For this review, use the dimensioned drawing (mm, ordinates from the lowest corner) and the shaded views. A direction names the side the tool comes from. Give positions to 0.01 mm unless a question says otherwise; leave off trailing zeros. Write each loop counter-clockwise with the first axis right and the second up, starting at its lowest first coordinate (ties: lowest second). Pieces come first, ordered by that corner, then holes. Notation, with made-up numbers: M 23,6 L 75,6 A35 ccw 75,45 Z; hole C -8,54.25 d2. An arc over 180 degrees is marked long. One line per item, written item: value. Start each with the question number.
Item 1: Clearance check with flat-ended pins moving along their axes: pin 1 Ø2.5 at (x, z) = (11, 29) entering from -Y; pin 2 Ø8 at (y, z) = (8, 21.5) entering from -X; pin 3 Ø1 at (x, y) = (11.5, 10) entering from +Z; pin 4 Ø1.5 at (y, z) = (9.5, 12.5) entering from +X. State where each tip first meets the part, or that it passes through.
Item 2: Consider section A-A, the plane z = 28.5. Write out the cut boundary in (x, y), and give its area (3 significant figures).
Item 3: Consider section C-C, the plane y = 4.5. Write out the cut boundary in (x, z).
Item 4: Consider section D-D, the plane x = 18. Write out the cut boundary in (y, z).
Item 5: Consider section B-B, the plane x = 35. Write out the cut boundary in (y, z), and give its area (3 significant figures).
Item 6: Tool access review of the marked faces 1, 2 and 3: name each direction out of +Z, -Z, +X, -X, +Y, -Y from which nothing blocks a thin tool from reaching the whole face with its end or side.
Item 7: Mouldability with a two-part tool opening along Y and no side actions: class the marked faces 4, 5 and 6 as released by +Y, released by -Y, zero draft, split by the parting line, or undercut.
Item 8: To check wall thickness, follow probe 1 along X at (y, z) = (10, 3.1); probe 2 along Y at (x, z) = (11, 25.5); probe 3 along Z at (x, y) = (16.9, 10). State the ranges of each line that lie inside material, in increasing order.
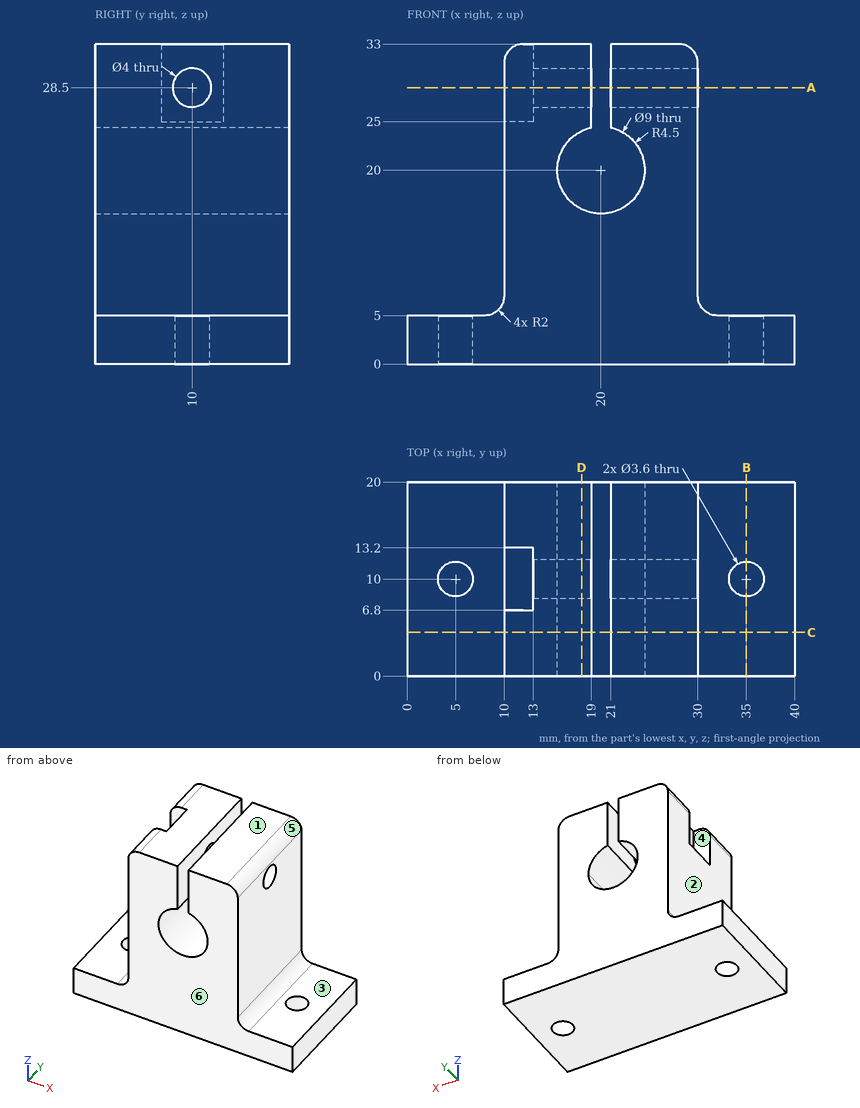
Model answer:
1. pin 1: stops at y = 0
1. pin 2: stops at x = 10
1. pin 3: stops at z = 25
1. pin 4: stops at x = 30
2. outline: M 10,0 L 19,0 L 19,8 L 13,8 L 13,6.8 L 10,6.8 Z; M 10,13.2 L 13,13.2 L 13,12 L 19,12 L 19,20 L 10,20 Z; M 21,0 L 30,0 L 30,8 L 21,8 Z; M 21,12 L 30,12 L 30,20 L 21,20 Z
2. area: 281 mm2
3. outline: M 0,0 L 40,0 L 40,5 L 32,5 A2 cw 30,7 L 30,31 A2 ccw 28,33 L 21,33 L 21,24.39 A4.5 cw long 19,24.39 L 19,33 L 12,33 A2 ccw 10,31 L 10,7 A2 cw 8,5 L 0,5 Z
4. outline: M 0,0 L 20,0 L 20,15.97 L 0,15.97 Z; M 0,24.03 L 20,24.03 L 20,33 L 0,33 Z; hole C 10,28.5 d4
5. outline: M 0,0 L 8.2,0 L 8.2,5 L 0,5 Z; M 11.8,0 L 20,0 L 20,5 L 11.8,5 Z
5. area: 82.0 mm2
6. face 1: +Z, +X, -X, +Y, -Y
6. face 2: +Z, -X, +Y, -Y
6. face 3: +Z, +X, +Y, -Y
7. face 4: undercut
7. face 5: zero draft
7. face 6: released by -Y
8. probe 1: x = 0 to 3.2, 6.8 to 33.2, 36.8 to 40
8. probe 2: y = 0 to 6.8, 13.2 to 20
8. probe 3: z = 0 to 16.74, 23.26 to 26.5, 30.5 to 33
